Autodesk Inventor part; units mm, degrees
ref_plane "YZ Plane" through (0, 0, 0) normal (1, 0, 0) x (0, 1, 0)
ref_plane "XZ Plane" through (0, 0, 0) normal (0, 1, 0) x (-1, 0, 0)
ref_plane "XY Plane" through (0, 0, 0) normal (0, 0, 1) x (1, 0, 0)
sketch "スケッチ1" plane through (0, 0, 0) normal (0, 0, 1) x (1, 0, 0)
  line L0 (-25, 35) -> (25, 35)
  line L1 (25, 35) -> (25, -35)
  line L2 (25, -35) -> (-25, -35)
  line L3 (-25, -35) -> (-25, 35)
  point P0 (0, 0)
  point P1 (-25, 0)
  point P2 (0, 35)
  dimension "d0" = 50
  dimension "d1" = 70
extrude "押し出し1" add sketch "スケッチ1" along normal blind 1.6
sketch "スケッチ2" plane through (0, 0, 1.6) normal (0, 0, 1) x (1, 0, 0)
  line L0 (-25, 35) -> (-25, -35)
  line L1 (-25, 8) -> (-3, 8)
  line L2 (-3, 8) -> (-3, -8)
  line L3 (-3, -8) -> (-25, -8)
  line L4 (-25, -8) -> (-25, 8)
  circle A0 centre (0, 0) radius 1.5
  point P0 (-25, 0)
  dimension "d10" = 16
  dimension "d11" = 3
  dimension "d12" = 25
  dimension "d13" = 3
extrude "押し出し2" cut sketch "スケッチ2" against normal through all
fillet "フィレット1" radius 20 2 edges at (-25, -35, 0.8) (-25, 35, 0.8)
sketch "スケッチ3" plane through (0, 0, 1.6) normal (0, 0, 1) x (1, 0, 0)
  line L0 (25, -35) -> (25, 35)
  line L1 (25, 35) -> (-5, 35)
  line L2 (-30.9592, 0) -> (30.9592, 0) construction
  line L3 (-25, 8) -> (-3, 8) construction
  line L4 (-25, 15) -> (-25, 8) construction
  point P0 (0, 0)
  point P1 (21, 0)
  point P2 (-21, -12)
  point P3 (5, -31)
  point P4 (5, 31)
  point P5 (0, 0)
  dimension "d26" = 30
  dimension "d27" = 4
  dimension "d28" = 4
hole "穴1" at (5, 31, 1.6) at (21, 0, 1.6) at (5, -31, 1.6) direction (0, 0, -1) diameter 3.2 end through all
properties part number "PCB-main"
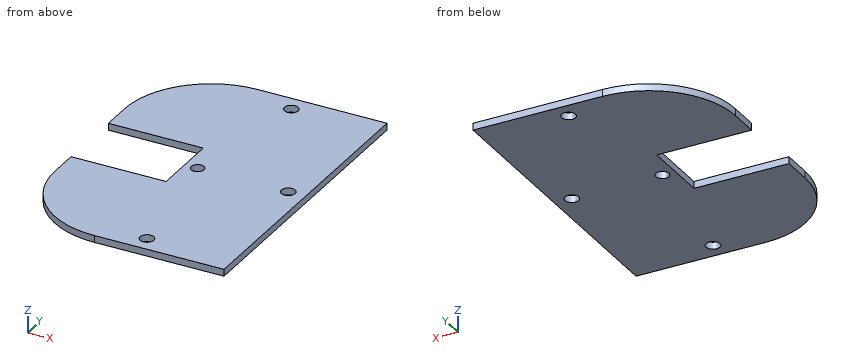
Part model, mm, in its own coordinate system. Coordinates: 2 decimals unless noted, no trailing zeros. Order: outer loops, then holes, each group sorted by start corner. A loop starts at its lowest first (then second) coordinate and runs counter-clockwise, first axis right, second up.
(1) Slice it at C-C, the plane z = 0.25. Write the cut outline in (x, y).
Check sheet entries:
outline: (-25, -15) arc R20 ccw to (-5, -35) - (25, -35) - (25, 35) - (-5, 35) arc R20 ccw to (-25, 15) - (-25, 8) - (-3, 8) - (-3, -8) - (-25, -8) - close; hole circle Ø3 at (0, 0); hole circle Ø3.2 at (5, -31); hole circle Ø3.2 at (5, 31); hole circle Ø3.2 at (21, 0)
(2) Pin check, flat tips, straight feed: pin 1 Ø0.5 at (y, z) = (-1, 1) entering from -X; pin 2 Ø0.5 at (x, z) = (-17.5, 0.5) entering from +Y. Stop position of each tip, or through.
Check sheet entries:
pin 1: stops at x = -3
pin 2: stops at y = 30.81
(3) Slice it at A-A, the plane x = 0. Write the cut outline in (y, z).
Check sheet entries:
outline: (-35, 0) - (-1.5, 0) - (-1.5, 1.6) - (-35, 1.6) - close; (1.5, 0) - (35, 0) - (35, 1.6) - (1.5, 1.6) - close
(4) Slice it at D-D, the plane y = 0. Write the cut outline in (x, z), and give its area (3 significant figures).
Check sheet entries:
outline: (-3, 0) - (-1.5, 0) - (-1.5, 1.6) - (-3, 1.6) - close; (1.5, 0) - (19.4, 0) - (19.4, 1.6) - (1.5, 1.6) - close; (22.6, 0) - (25, 0) - (25, 1.6) - (22.6, 1.6) - close
area: 34.9 mm2
(5) Slice it at B-B, the plane y = -31. Write the cut outline in (x, z), and give its area (3 significant figures).
Check sheet entries:
outline: (-17, 0) - (3.4, 0) - (3.4, 1.6) - (-17, 1.6) - close; (6.6, 0) - (25, 0) - (25, 1.6) - (6.6, 1.6) - close
area: 62.1 mm2
(6) Probe L1, parallel to Y at x = 5, z = 0.6; L2, parallel to Y at x = 4.5, z = 0.9; L3, parallel to Y at x = 0, z = 1.15. List the from-to ranges inside material, lowest first.
Check sheet entries:
L1: y = -35 to -32.6, -29.4 to 29.4, 32.6 to 35
L2: y = -35 to -32.52, -29.48 to 29.48, 32.52 to 35
L3: y = -35 to -1.5, 1.5 to 35
